from build123d import *

# Parameters (mm, degrees)
F1_DEPTH = 100
F2_R     = 8


with BuildPart() as f1:
    # F0 (on Top) → F1 (new body)
    with BuildSketch(Plane.XY):
        Polygon((-43, 25), (-50, 25), (-50, -25), (-43, -25), (-43, -2.5), (43, -2.5), (43, -25), (50, -25), (50, 25), (43, 25), (43, 2.5), (-43, 2.5), align=None)
    extrude(amount=F1_DEPTH)

    # F2
    f2_edges = [f1.edges().sort_by_distance(p)[0] for p in [
        (43, -2.5, 50),
        (-43, -2.5, 50),
        (-43, 2.5, 50),
        (43, 2.5, 50),
    ]]
    fillet(f2_edges, radius=F2_R)


solid = f1.part
The listing builds one solid part. Answer for the finished solid, in the listing's coordinates (mm). A direction names the side the tool comes from. Round coordinates to 2 decimals unless told otherwise and drop trailing zeros. Write each loop counter-clockwise with the first axis right and the second up, starting at its lowest first coordinate (ties: lowest second). Pieces come first, ordered by that corner, then holes. Notation, with made-up numbers: M 83.5,3 L 116.5,3 A12 cw 116.5,7 Z; hole C 2.25,19.25 d3. An arc over 180 degrees is marked long. Write each question's results on one line, items separated by ' | '. Start each with the question number.
Item 1: Straight lines are drawn through the part: L1, parallel to X at y = -20, z = 4; L2, parallel to Y at x = -0.5, z = 78.5; L3, parallel to X at y = 4, z = 45.5. For each, find the intervals that lie inside material, in ascending order. Write a range as [from, to].
Item 2: A cutting plane is placed at A-A on y = -15. Write down the section's boundary in (x, z), and give its area (3 significant figures).
Item 3: A cutting plane is placed at D-D on y = 8.5. Write down the section's boundary in (x, z).
Item 4: For faces 4 (the face through (40.719, 4.906, 50.7)), 5 (the face through (-40.719, -4.906, 50.7)), 6 (the face through (46, -25, 49)), determine the directions among +Z, -Z, +X, -X, +Y, -Y from which every point of the face is accessible in a straight line to the end or side of a thin tool.
Item 5: A cutting plane is placed at B-B on z = 73.5. Write down the section's boundary in (x, y).
Item 6: A cutting plane is placed at C-C on x = -21. Write down the section's boundary in (y, z), and give its area (3 significant figures).
Item 7: For a pull along X with two mould halves and no side action, classify faces 1 (the face through (50, 0, 49)), 2 (the face through (-43, -18, 49)), 3 (the face through (-47, -25, 49)) as pulls with the +X half, pulls with the -X half, needs draft (parallel to the pull), parting line crosses it, or undercut.
Item 8: Flat-ended cylindrical pins translate along their axes: pin 1 Ø5 at (x, z) = (25, 85.5) entering from +Y; pin 2 Ø5 at (x, z) = (33.5, 60) entering from +Y; pin 3 Ø6 at (x, z) = (17, 84.5) entering from -Y. Find the tip coordinate at first contact, or state that the pin passes through.
Check sheet entries:
1) L1: [-50, -43], [43, 50] | L2: [-2.5, 2.5] | L3: [-50, -39.66], [39.66, 50]
2) outline: M -50,0 L -43,0 L -43,100 L -50,100 Z; M 43,0 L 50,0 L 50,100 L 43,100 Z | area: 1,400 mm²
3) outline: M -50,0 L -42.75,0 L -42.75,100 L -50,100 Z; M 42.75,0 L 50,0 L 50,100 L 42.75,100 Z
4) face 4: +Z, -Z, +Y | face 5: +Z, -Z, -Y | face 6: +Z, -Z, +X, -X, -Y
5) outline: M -50,-25 L -43,-25 L -43,-10.5 A8 cw -35,-2.5 L 35,-2.5 A8 cw 43,-10.5 L 43,-25 L 50,-25 L 50,25 L 43,25 L 43,10.5 A8 cw 35,2.5 L -35,2.5 A8 cw -43,10.5 L -43,25 L -50,25 Z
6) outline: M -2.5,0 L 2.5,0 L 2.5,100 L -2.5,100 Z | area: 500 mm²
7) face 1: pulls with the +X half | face 2: undercut | face 3: needs draft
8) pin 1: y = 2.5 | pin 2: y = 2.56 | pin 3: y = -2.5
